Read the model definition and answer for the solid it produces. Units are mm, in the model's axes. Face numbers are marked on the shaded views. A direction names the side the tool comes from. Coordinates: 2 decimals unless noted, no trailing zeros. Loops run counter-clockwise (first coordinate to the right, second up) from the corner with the lowest first, then second, coordinate; pieces in that order, holes last. Notation, with made-up numbers: (50, 29.25) - (89, 29.25) arc R20 ccw to (89, 67.25) - close; hole circle Ø1 at (59.5, 67.5). An arc over 180 degrees is marked (long way). Use CSV: the item, a comma, the result in double quotes.
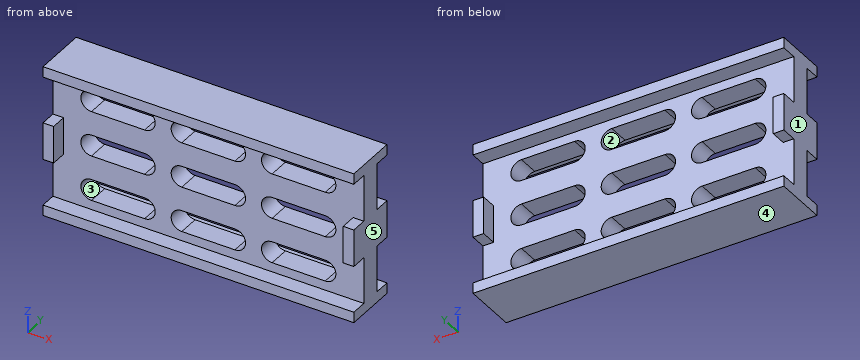
```python
from build123d import *

# Parameters (mm, degrees)
SKETCH1_W           = 54.5
SKETCH1_H           = 24.5
BOSS_EXTRUDE1_DEPTH = 2
BOSS_EXTRUDE2_START = -2
SKETCH2_W           = 58.5
SKETCH2_H           = 28.5
SKETCH2_W_2         = 54.5
SKETCH2_H_2         = 24.5
BOSS_EXTRUDE2_DEPTH = 5
CUT_EXTRUDE1_DEPTH  = 33.918459867
FILL_PATTERN1_DEPTH = 2
LPATTERN1_COUNT     = 2
LPATTERN1_PITCH     = 8.5
LPATTERN1_COL_COUNT = 2
LPATTERN1_COL_PITCH = 8.5
SKETCH13_W          = 8.75
SKETCH13_H          = 3
CUT_EXTRUDE2_DEPTH  = 61.417816081


# Read off the part's stored shape, not the designer's step: Fill Pattern1
with BuildPart() as part:
    # Sketch1 → Boss-Extrude1 (new body)
    with BuildSketch(Plane(origin=(0, 0, 0), x_dir=(1, 0, 0), z_dir=(0, 1, 0))):
        Rectangle(SKETCH1_W, SKETCH1_H)
    extrude(amount=BOSS_EXTRUDE1_DEPTH)

    # Sketch2 → Boss-Extrude2 (add)
    with BuildSketch(Plane(origin=(0, 2, 0), x_dir=(1, 0, 0), z_dir=(0, 1, 0)).offset(BOSS_EXTRUDE2_START)):
        Rectangle(SKETCH2_W, SKETCH2_H)
        Rectangle(SKETCH2_W_2, SKETCH2_H_2, mode=Mode.SUBTRACT)
    extrude(amount=BOSS_EXTRUDE2_DEPTH)

    # Sketch5 → Cut-Extrude1 (cut, through all)
    with BuildSketch(Plane.XZ):
        with BuildLine():
            Line((-5, 2), (5, 2))
            ThreePointArc((5, 2), (7, 0), (5, -2))
            Line((5, -2), (-5, -2))
            ThreePointArc((-5, -2), (-7, 0), (-5, 2))
        make_face()
    cut_extrude1 = extrude(amount=-CUT_EXTRUDE1_DEPTH, mode=Mode.SUBTRACT)

    # Fill Pattern1 outline → Fill Pattern1 (cut)
    with BuildSketch(Plane(origin=(0, 0, 0), x_dir=(1, 0, 0), z_dir=(0, 1, 0))):
        with BuildLine():
            ThreePointArc((-22, 2), (-24, 0), (-22, -2))
            Line((-22, -2), (-12, -2))
            ThreePointArc((-12, -2), (-10, 0), (-12, 2))
            Line((-12, 2), (-22, 2))
        make_face()
        with BuildLine():
            ThreePointArc((12, 2), (10, 0), (12, -2))
            Line((12, -2), (22, -2))
            ThreePointArc((22, -2), (24, 0), (22, 2))
            Line((22, 2), (12, 2))
        make_face()
        with BuildLine():
            ThreePointArc((-22, 10.5), (-24, 8.5), (-22, 6.5))
            Line((-22, 6.5), (-12, 6.5))
            ThreePointArc((-12, 6.5), (-10, 8.5), (-12, 10.5))
            Line((-12, 10.5), (-22, 10.5))
        make_face()
        with BuildLine():
            ThreePointArc((12, 10.5), (10, 8.5), (12, 6.5))
            Line((12, 6.5), (22, 6.5))
            ThreePointArc((22, 6.5), (24, 8.5), (22, 10.5))
            Line((22, 10.5), (12, 10.5))
        make_face()
        with BuildLine():
            ThreePointArc((-22, -6.5), (-24, -8.5), (-22, -10.5))
            Line((-22, -10.5), (-12, -10.5))
            ThreePointArc((-12, -10.5), (-10, -8.5), (-12, -6.5))
            Line((-12, -6.5), (-22, -6.5))
        make_face()
        with BuildLine():
            ThreePointArc((12, -6.5), (10, -8.5), (12, -10.5))
            Line((12, -10.5), (22, -10.5))
            ThreePointArc((22, -10.5), (24, -8.5), (22, -6.5))
            Line((22, -6.5), (12, -6.5))
        make_face()
    extrude(amount=FILL_PATTERN1_DEPTH, mode=Mode.SUBTRACT)

    # LPattern1: Cut-Extrude1 ×2
    with Locations(*[(0, 0, i * LPATTERN1_PITCH) for i in range(1, LPATTERN1_COUNT)]):
        add(cut_extrude1, mode=Mode.SUBTRACT)

    # LPattern1 col: Cut-Extrude1 ×2
    with Locations(*[(0, 0, -i * LPATTERN1_COL_PITCH) for i in range(1, LPATTERN1_COL_COUNT)]):
        add(cut_extrude1, mode=Mode.SUBTRACT)

    # Sketch13 → Cut-Extrude2 (cut, through all)
    with BuildSketch(Plane(origin=(29.25, 0, 0), x_dir=(0, 0, -1), z_dir=(1, 0, 0))):
        with Locations((-7.875, 3.5)):
            Rectangle(SKETCH13_W, SKETCH13_H)
        with Locations((7.875, 3.5)):
            Rectangle(SKETCH13_W, SKETCH13_H)
    extrude(amount=-CUT_EXTRUDE2_DEPTH, mode=Mode.SUBTRACT)

    # Mirror1: part across plane


with BuildPart() as part_1:
    add(part.part)
    add(part.part.mirror(Plane(origin=(0, 0, 0), x_dir=(0, 0, 1), z_dir=(0, -1, 0))))


solid = part_1.part
```
Q1. The part is cut by section D-D on z = 0. Determine the outline of the cut face in (x, y), and give its area (3 significant figures).
Reported:
outline,"(-29.25, -5) - (-27.25, -5) - (-27.25, -2) - (-24, -2) - (-24, 2) - (-27.25, 2) - (-27.25, 5) - (-29.25, 5) - close; (-10, -2) - (-7, -2) - (-7, 2) - (-10, 2) - close; (7, -2) - (10, -2) - (10, 2) - (7, 2) - close; (24, -2) - (27.25, -2) - (27.25, -5) - (29.25, -5) - (29.25, 5) - (27.25, 5) - (27.25, 2) - (24, 2) - close"
area,"90.0 mm²"
Q2. The part is cut by section A-A on y = 3. Determine the outline of the cut face in (x, z).
Reported:
outline,"(-29.25, -14.25) - (29.25, -14.25) - (29.25, -12.25) - (-29.25, -12.25) - close; (-29.25, -3.5) - (-27.25, -3.5) - (-27.25, 3.5) - (-29.25, 3.5) - close; (-29.25, 12.25) - (29.25, 12.25) - (29.25, 14.25) - (-29.25, 14.25) - close; (27.25, -3.5) - (29.25, -3.5) - (29.25, 3.5) - (27.25, 3.5) - close"
Q3. Find the intervals of material crossed by probe 1 along Z at (x, y) = (-15.5, 1); probe 2 along X at (y, z) = (4.5, -2); probe 3 along Z at (x, y) = (-14.5, 3.75), in increasing order. Write a range as [from, to].
Reported:
probe 1,"z = [-14.25, -10.5], [-6.5, -2], [2, 6.5], [10.5, 14.25]"
probe 2,"x = [-29.25, -27.25], [27.25, 29.25]"
probe 3,"z = [-14.25, -12.25], [12.25, 14.25]"
Q4. Given P1, Ø8, axis at x = 21, z = 1, coming from the +Y side; P2, Ø8, axis at x = -20.5, z = -5, coming from the -Y side, each flat-ended and moving along its own axis, determine where each tip first touches the part or whether it passes through.
Reported:
P1,"stops at y = 2"
P2,"stops at y = -2"
Q5. The part is cut by section C-C on x = -15. Determine the outline of the cut face in (y, z).
Reported:
outline,"(-5, -14.25) - (5, -14.25) - (5, -12.25) - (2, -12.25) - (2, -10.5) - (-2, -10.5) - (-2, -12.25) - (-5, -12.25) - close; (-5, 12.25) - (-2, 12.25) - (-2, 10.5) - (2, 10.5) - (2, 12.25) - (5, 12.25) - (5, 14.25) - (-5, 14.25) - close; (-2, -6.5) - (2, -6.5) - (2, -2) - (-2, -2) - close; (-2, 2) - (2, 2) - (2, 6.5) - (-2, 6.5) - close"
Q6. The part is cut by section B-B on z = -8.5. Determine the outline of the cut face in (x, y).
Reported:
outline,"(-29.25, -2) - (-24, -2) - (-24, 2) - (-29.25, 2) - close; (-10, -2) - (-7, -2) - (-7, 2) - (-10, 2) - close; (7, -2) - (10, -2) - (10, 2) - (7, 2) - close; (24, -2) - (29.25, -2) - (29.25, 2) - (24, 2) - close"
Q7. A tool of negligible diameter and unlimited length cuts with its end or side. For the marked faces 1 and 2, from which of +Z, -Z, +X, -X, +Y, -Y can it reach the whole face along a straight path? Write none if from no direction.
Reported:
face 1,"+Z, -Z, -X, +Y, -Y"
face 2,"+Y, -Y"
Q8. For a pull along X with two mould halves and no side action, classify the marked faces 3, 4 and 5 as +X half, -X half, draft (parallel to the pull), parting line (faces both ways), or undercut.
Reported:
face 3,"undercut"
face 4,"draft"
face 5,"+X half"
